```python
from build123d import *

# Parameters (mm, degrees)
BOSS_EXTRUDE1_DEPTH = 61.722
SKETCH3_R           = 17.5006
CUT_EXTRUDE1_DEPTH  = 9.906
SKETCH4_R           = 14.9606
CUT_EXTRUDE2_DEPTH  = 147.78694942
SKETCH5_R           = 3.175
CUT_EXTRUDE3_DEPTH  = 157.380066773
SKETCH6_R           = 17.5006
CUT_EXTRUDE4_DEPTH  = 9.906
SKETCH7_R           = 14.9606
CUT_EXTRUDE5_DEPTH  = 147.78694942
FILLET1_R           = 1.27


with BuildPart() as part:
    # Sketch2 → Boss-Extrude1 (new body)
    with BuildSketch(Plane(origin=(0, 0, 0), x_dir=(1, 0, 0), z_dir=(0, 1, 0))):
        Polygon((0, 0), (0, 101.6), (-101.6, 101.6), (-101.6, 76.2), (-25.4, 76.2), (-25.4, 0), align=None)
    extrude(amount=BOSS_EXTRUDE1_DEPTH)

    # Sketch3 → Cut-Extrude1 (cut)
    with BuildSketch(Plane.XY.offset(-76.2)):
        with Locations((-64.1604, 30.861)):
            Circle(SKETCH3_R)
    extrude(amount=-CUT_EXTRUDE1_DEPTH, mode=Mode.SUBTRACT)

    # Sketch4 → Cut-Extrude2 (cut, through all)
    with BuildSketch(Plane.XY.offset(-86.106)):
        with Locations((-64.1604, 30.861)):
            Circle(SKETCH4_R)
    extrude(amount=-CUT_EXTRUDE2_DEPTH, mode=Mode.SUBTRACT)

    # Sketch5 → Cut-Extrude3 (cut, through all)
    with BuildSketch(Plane(origin=(0, 61.722, 0), x_dir=(1, 0, 0), z_dir=(0, 1, 0))):
        with Locations(Location((-88.9, 88.9, 0), (0, 0, 270))):
            Circle(SKETCH5_R)
        with Locations(Location((-12.7, 88.9, 0), (0, 0, 270))):
            Circle(SKETCH5_R)
        with Locations(Location((-12.7, 12.7, 0), (0, 0, 270))):
            Circle(SKETCH5_R)
    extrude(amount=-CUT_EXTRUDE3_DEPTH, mode=Mode.SUBTRACT)

    # Sketch6 → Cut-Extrude4 (cut)
    with BuildSketch(Plane.ZY.offset(25.4)):
        with Locations((-37.4396, 30.861)):
            Circle(SKETCH6_R)
    extrude(amount=-CUT_EXTRUDE4_DEPTH, mode=Mode.SUBTRACT)

    # Sketch7 → Cut-Extrude5 (cut, through all)
    with BuildSketch(Plane.ZY.offset(15.494)):
        with Locations((-37.4396, 30.861)):
            Circle(SKETCH7_R)
    extrude(amount=-CUT_EXTRUDE5_DEPTH, mode=Mode.SUBTRACT)

    # Fillet1
    fillet1_edges = [part.edges().sort_by_distance(p)[0] for p in [
        (-25.4, 30.861, 0),
        (-25.4, 30.861, -76.2),
        (-101.6, 30.861, -76.2),
        (-101.6, 30.861, -101.6),
        (0, 30.861, -101.6),
        (0, 30.861, 0),
        (-50.8, 61.722, -101.6),
        (-101.6, 61.722, -88.9),
        (-63.5, 61.722, -76.2),
        (-25.4, 61.722, -38.1),
        (-12.7, 61.722, 0),
        (-25.4, 0, -38.1),
        (-63.5, 0, -76.2),
        (-101.6, 0, -88.9),
        (-50.8, 0, -101.6),
        (0, 0, -50.8),
        (-12.7, 0, 0),
        (0, 61.722, -50.8),
    ]]
    fillet(fillet1_edges, radius=FILLET1_R)


solid = part.part
```
CAD build for the part. Positions are in the model's coordinates, mm. A direction names the side the tool comes from. Round coordinates to 2 decimals unless told otherwise and drop trailing zeros. Loops run counter-clockwise (first coordinate to the right, second up) from the corner with the lowest first, then second, coordinate; pieces in that order, holes last. Notation, with made-up numbers: M 10.5,12 L 26.5,12 A8 cw 26.5,24 Z; hole C 17,85.5 d8. An arc over 180 degrees is marked long. Use a Markdown table: item, result. Add a question column.
(1) Drill centre lines: line 1 (Z direction, x = -13.5, y = 40); line 2 (X direction, y = 52.5, z = -56.5); line 3 (Z direction, x = -51.5, y = 11). Where is each one in solid material? Low to high.
(2) Cut at A-A (z = -12.7). Give the cut face in (x, y) (3 decimals).
(3) Cut at D-D (y = 36.5). State how many separate pieces and enclosed holes the cut face has, and give its area (3 significant figures).
(4) Pull direction Y, two halves, no side cores. Call faces 5 (the face through (-7.855, 45.694, -39.387)), 6 (the face through (-88.76, 31.29, -92.07)), 7 (the face through (-29, 61.722, -85)): +Y half, -Y half, draft (parallel to the pull), parting line (faces both ways), or undercut.
(5) Cut at C-C (x = -67). Give the cut face in (y, z).
(6) Flat gauge pins, fed straight in: pin 1 (17.5 mm diameter, centred on y = 31.5, z = -45.5, fed in from -X); pin 2 (18 mm diameter, centred on x = -49, y = 34, fed in from +Z); pin 3 (10 mm diameter, centred on x = -12.7, z = -12.7, fed in from -Y). Where does each tip first touch, or does it go through?
(7) Cut at B-B (y = 50). Give the cut face in (x, z) (3 decimals).
(8) Which spindle directions (+Z, -Z, +X, -X, +Y, -Y) get a long thin tool onto all of the face, cutting with end or side? Do faces 1 (the face through (-47.6, 23.9, -76.2)), 2 (the face through (-51, 39, -86.106)), 3 (the face through (-20.516, 13.777, -41.233)), 4 (the face through (-13, 30, 0)). Say none if no direction does.
Geometry says:
| question | item | result |
|---|---|---|
| 1 | line 1 | z = -101.6 to -91.97, -85.83 to -49.28, -25.59 to -15.77, -9.63 to 0 |
| 1 | line 2 | x = -25.4 to 0 |
| 1 | line 3 | z = -101.6 to -76.2 |
| 2 | outline | M -25.4,1.27 A1.27 ccw -24.13,0 L -15.875,0 L -15.875,61.722 L -24.13,61.722 A1.27 ccw -25.4,60.452 Z; M -9.525,0 L -1.27,0 A1.27 ccw 0,1.27 L 0,60.452 A1.27 ccw -1.27,61.722 L -9.525,61.722 Z |
| 3 | separate pieces | 3 |
| 3 | enclosed holes | 3 |
| 3 | area | 2,900 mm² |
| 4 | face 5 | undercut |
| 4 | face 6 | draft |
| 4 | face 7 | +Y half |
| 5 | outline | M 0,-100.33 A1.27 ccw 1.27,-101.6 L 16.17,-101.6 L 16.17,-86.11 L 13.59,-86.11 L 13.59,-76.2 L 1.27,-76.2 A1.27 ccw 0,-77.47 Z; M 45.55,-101.6 L 60.45,-101.6 A1.27 ccw 61.72,-100.33 L 61.72,-77.47 A1.27 ccw 60.45,-76.2 L 48.13,-76.2 L 48.13,-86.11 L 45.55,-86.11 Z |
| 6 | pin 1 | stops at x = -15.49 |
| 6 | pin 2 | stops at z = -76.2 |
| 6 | pin 3 | stops at y = 0 |
| 7 | outline | M -101.6,-100.33 A1.27 ccw -100.33,-101.6 L -1.27,-101.6 A1.27 ccw 0,-100.33 L 0,-1.27 A1.27 ccw -1.27,0 L -24.13,0 A1.27 ccw -25.4,-1.27 L -25.4,-74.93 A1.27 cw -26.67,-76.2 L -100.33,-76.2 A1.27 ccw -101.6,-77.47 Z; hole C -88.9,-88.9 d6.35; hole C -12.7,-88.9 d6.35; hole C -12.7,-12.7 d6.35 |
| 8 | face 1 | +Z, -X, +Y, -Y |
| 8 | face 2 | +Z |
| 8 | face 3 | -X |
| 8 | face 4 | +Z, +X, -X, +Y, -Y |
